Geometry: final body of the model. Coordinates: model frame, mm. Face numbers are marked on the shaded views. A direction names the side the tool comes from. Coordinates: 2 decimals unless noted, no trailing zeros. Write each loop counter-clockwise with the first axis right and the second up, starting at its lowest first coordinate (ties: lowest second). Pieces come first, ordered by that corner, then holes. Notation, with made-up numbers: (-23.5, 68.5) - (0.5, 68.5) arc R22 ccw to (0.5, 90.5) - close; hole circle Ø2 at (60, -23). An arc over 180 degrees is marked (long way). Answer as a JSON object with one key per item and string values. Group by question number.
Item 1: First-contact query: pin 1 Ø1 at (x, y) = (-5.5, -23) entering from +Z; pin 2 Ø3 at (y, z) = (14.5, 22) entering from +X. Flat tips, straight axial feed; report the tip coordinate or a pass-through.
Item 2: Line query: line 1 along X through (y, z) = (-25.4, 10.25); line 2 along Y through (x, z) = (-25.4, 6.5); line 3 along X through (y, z) = (-23.5, 20). Output: solid intervals per line, ascending. Write a range as from..to.
Item 3: Mould query, pull axis Z, two halves, no side actions, for the marked faces 1, 2, 3 and 4. Classes: pulls with the +Z half, pulls with the -Z half, needs draft (parallel to the pull), parting line crosses it, or undercut.
Item 4: Set-up query: the marked faces 5, 6 and 7. Return all of +Z, -Z, +X, -X, +Y, -Y with unobstructed straight access to the full face (end or side cutting, diameter ignored); none if empty.
Item 5: Section A-A on z = 15. State how many separate pieces and enclosed holes the cut face has, and give its area (3 significant figures).
Item 6: Section C-C on x = 35. Return loops of the section in (y, z), and give its area (3 significant figures).
Item 7: Section B-B on y = -21.5. Return loops of the section in (x, z).
```python
from build123d import *

# Parameters (mm, degrees)
SKETCH1_W                   = 60
SKETCH1_H                   = 62
BOSS_EXTRUDE1_DEPTH         = 30
SKETCH3_R                   = 7.5
BOSS_EXTRUDE2_DEPTH         = 25.5
SKETCH4_R                   = 15
BOSS_EXTRUDE3_DEPTH         = 15
FILLET1_R                   = 3
SKETCH1_3_W                 = 60
SKETCH1_3_H                 = 62
SKETCH1_3_R                 = 3.175
BOSS_EXTRUDE4_DEPTH         = 20
F_1_4_20_TAPPED_HOLE1_D     = 5.1054
F_1_4_20_TAPPED_HOLE1_DEPTH = 16.51
F_1_4_20_TAPPED_HOLE1_TIP   = 1.533816902
F_1_4_20_TAPPED_HOLE2_D     = 5.1054
F_1_4_20_TAPPED_HOLE2_DEPTH = 16.51
F_1_4_20_TAPPED_HOLE2_TIP   = 1.533816902
CUT_EXTRUDE1_DEPTH          = 63


with BuildPart() as part:
    # Sketch1 → Boss-Extrude1 (new body)
    with BuildSketch(Plane.XY):
        Rectangle(SKETCH1_W, SKETCH1_H)
    extrude(amount=BOSS_EXTRUDE1_DEPTH)

    # Sketch3 → Boss-Extrude2 (add)
    with BuildSketch(Plane(origin=(30, 0, 0), x_dir=(0, 0, -1), z_dir=(1, 0, 0))):
        with Locations((-15, 0)):
            Circle(SKETCH3_R)
    extrude(amount=BOSS_EXTRUDE2_DEPTH)

    # Sketch4 → Boss-Extrude3 (add)
    with BuildSketch(Plane(origin=(55.5, 0, 0), x_dir=(0, 0, -1), z_dir=(1, 0, 0))):
        with Locations((-15, 0)):
            Circle(SKETCH4_R)
    extrude(amount=BOSS_EXTRUDE3_DEPTH)

    # Fillet1
    fillet1_edges = [part.edges().sort_by_distance(p)[0] for p in [
        (55.5, 0, 30),
        (70.5, 0, 30),
    ]]
    fillet(fillet1_edges, radius=FILLET1_R)

    # Sketch1<3> → Boss-Extrude4 (add)
    with BuildSketch(Plane.XY):
        Rectangle(SKETCH1_3_W, SKETCH1_3_H)
        Circle(SKETCH1_3_R, mode=Mode.SUBTRACT)
        with Locations((25.4, 25.4)):
            Circle(SKETCH1_3_R, mode=Mode.SUBTRACT)
        with Locations((-25.4, 25.4)):
            Circle(SKETCH1_3_R, mode=Mode.SUBTRACT)
        with Locations((-25.4, -25.4)):
            Circle(SKETCH1_3_R, mode=Mode.SUBTRACT)
        with Locations((25.4, -25.4)):
            Circle(SKETCH1_3_R, mode=Mode.SUBTRACT)
        with Locations((-12.7, 12.7)):
            Circle(SKETCH1_3_R, mode=Mode.SUBTRACT)
        with Locations((12.7, 12.7)):
            Circle(SKETCH1_3_R, mode=Mode.SUBTRACT)
        with Locations((-12.7, -12.7)):
            Circle(SKETCH1_3_R, mode=Mode.SUBTRACT)
        with Locations((12.7, -12.7)):
            Circle(SKETCH1_3_R, mode=Mode.SUBTRACT)
    extrude(amount=BOSS_EXTRUDE4_DEPTH)

    # 1/4-20 Tapped Hole1
    with Locations(Plane(origin=(0, 0, 0), x_dir=(-1, 0, 0), z_dir=(0, 0, -1))):
        with Locations((-25.4, 25.4), (25.4, 25.4), (25.4, -25.4), (-25.4, -25.4)):
            Hole(F_1_4_20_TAPPED_HOLE1_D / 2, depth=F_1_4_20_TAPPED_HOLE1_DEPTH)
            with Locations((0, 0, -(F_1_4_20_TAPPED_HOLE1_DEPTH + F_1_4_20_TAPPED_HOLE1_TIP / 2))):  # 118° drill point
                Cone(0, F_1_4_20_TAPPED_HOLE1_D / 2, F_1_4_20_TAPPED_HOLE1_TIP, mode=Mode.SUBTRACT)

    # 1/4-20 Tapped Hole2
    with Locations(Plane(origin=(0, 0, 0), x_dir=(-1, 0, 0), z_dir=(0, 0, -1))):
        with Locations((-12.7, 12.7), (0, 0), (12.7, 12.7), (12.7, -12.7), (-12.7, -12.7)):
            Hole(F_1_4_20_TAPPED_HOLE2_D / 2, depth=F_1_4_20_TAPPED_HOLE2_DEPTH)
            with Locations((0, 0, -(F_1_4_20_TAPPED_HOLE2_DEPTH + F_1_4_20_TAPPED_HOLE2_TIP / 2))):  # 118° drill point
                Cone(0, F_1_4_20_TAPPED_HOLE2_D / 2, F_1_4_20_TAPPED_HOLE2_TIP, mode=Mode.SUBTRACT)

    # Sketch16 → Cut-Extrude1 (cut, through all)
    with BuildSketch(Plane.XZ.offset(31)):
        Polygon((-4.91, 24.72), (-19.57, 24.72), (-15.4, 30), (15.4, 30), (19.57, 24.72), (4.91, 24.72), (4.91, 18.9), (-4.91, 18.9), align=None)
    extrude(amount=-CUT_EXTRUDE1_DEPTH, mode=Mode.SUBTRACT)


solid = part.part
```
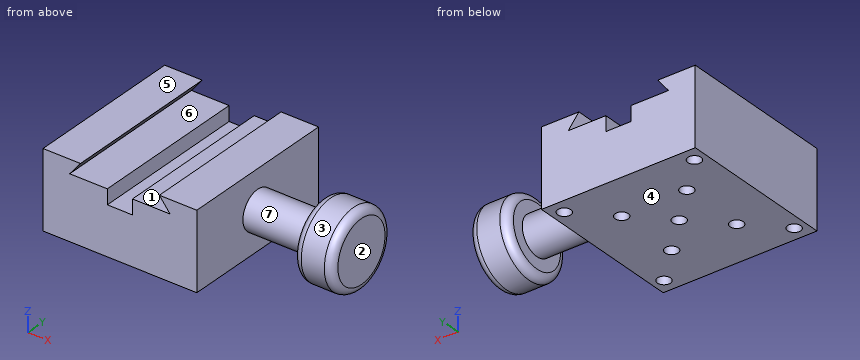
Checks:
{
 "1": {"pin 1": "z = 24.72", "pin 2": "x = 68.99"},
 "2": {"line 1": "-30..-27.95, -22.85..22.85, 27.95..30", "line 2": "-31..-27.95, -22.85..22.85, 27.95..31", "line 3": "-30..-4.91, 4.91..30"},
 "3": {"face 1": "undercut", "face 2": "needs draft", "face 3": "parting line crosses it", "face 4": "pulls with the -Z half"},
 "4": {"face 5": "+Z, +X, -X, +Y, -Y", "face 6": "+Y, -Y", "face 7": "none"},
 "5": {"separate pieces": "1", "enclosed holes": "9", "area": "4,360 mm^2"},
 "6": {"outline": "circle Ø15 at (0, 15)", "area": "177 mm^2"},
 "7": {"outline": "(-30, 0) - (30, 0) - (30, 30) - (15.4, 30) - (19.57, 24.72) - (4.91, 24.72) - (4.91, 18.9) - (-4.91, 18.9) - (-4.91, 24.72) - (-19.57, 24.72) - (-15.4, 30) - (-30, 30) - close"}
}
